Here's how the part is built. I have some questions about the finished solid (model axes, mm). Face numbers are marked on the shaded views. A direction names the side the tool comes from. Coordinates: 2 decimals unless noted, no trailing zeros. Order: outer loops, then holes, each group sorted by start corner. A loop starts at its lowest first (then second) coordinate and runs counter-clockwise, first axis right, second up. Notation, with made-up numbers: (77, 64.5) - (82, 64.5) arc R29 ccw to (82, 103.5) - close; hole circle Ø4 at (-9, -33). An arc over 180 degrees is marked (long way). Answer as CSV lines item,"result". Start each with the question number.
Q1. Suppose I cut it at D-D (y = -0.5). Please give me the cut outline in (x, z), then the cut area to 3 significant figures.
Q2. For the marked faces 1 and 2, which set-ups out of +Z, -Z, +X, -X, +Y, -Y let a thin tool reach every point of the face, with its end or its side?
Q3. For pin 1 Ø0.8 at (x, y) = (-17, 59.5) entering from +Z; pin 2 Ø4 at (x, z) = (33, 14) entering from +Y; pin 3 Ø2.5 at (y, z) = (60, -5) entering from +X, each with a flat end and sliding along its axis, tell me the tip position at first contact or that it passes through.
Q4. I need wall thicknesses on line 1 (X direction, y = 6, z = 3); line 2 (Z direction, x = -16, y = 4). Which ranges of each line are inside material? Lowest first, please.
Q5. Suppose I cut it at B-B (x = 18.3). Please give me the cut outline in (y, z), then the cut area to 3 significant figures.
Q6. Thinking about a two-plate mould opening in X: for the marked faces 3, 4 and 5, which applies, released by +X, released by -X, zero draft, split by the parting line, or undercut?
Q7. Suppose I cut it at A-A (z = 11.5). Please give me the cut outline in (x, y).
Q8. Suppose I cut it at C-C (z = -4). Please give me the cut outline in (x, y).
Autodesk Inventor part; units mm, degrees
ref_plane "YZ Plane" through (0, 0, 0) normal (1, 0, 0) x (0, 1, 0)
ref_plane "XZ Plane" through (0, 0, 0) normal (0, 1, 0) x (-1, 0, 0)
ref_plane "XY Plane" through (0, 0, 0) normal (0, 0, 1) x (1, 0, 0)
sketch "Sketch1" plane through (0, 0, 0) normal (0, 0, 1) x (1, 0, 0)
  line L0 (-42.25, 42.25) -> (42.25, 42.25)
  line L1 (42.25, 42.25) -> (42.25, -42.25)
  line L2 (42.25, -42.25) -> (-42.25, -42.25)
  line L3 (-42.25, -42.25) -> (-42.25, 42.25)
  line L4 (-42.25, 42.25) -> (42.25, -42.25) construction
  line L5 (42.25, 42.25) -> (-42.25, -42.25) construction
  line L6 (-45, 45) -> (45, 45)
  line L7 (45, 45) -> (45, -45)
  line L8 (45, -45) -> (-45, -45)
  line L9 (-45, -45) -> (-45, 45)
  line L10 (-45, 45) -> (45, -45) construction
  line L11 (45, 45) -> (-45, -45) construction
  point P0 (0, 0)
  dimension "d0" = 84.5
  dimension "d1" = 84.5
  dimension "d2" = 90
  dimension "d3" = 90
extrude "Extrusion1" add sketch "Sketch1" along normal blind 18
extrude "Extrusion2" add sketch "Sketch1" against normal blind 8 contours L0 L1 L2 L3 | L6 L7 L8 L9
sketch "Sketch2" plane through (0, 0, 18) normal (0, 0, 1) x (1, 0, 0)
  line L0 (42.25, -42.25) -> (42.25, 42.25)
  line L1 (42.25, 42.25) -> (-42.25, 42.25)
  line L2 (-42.25, 42.25) -> (-42.25, -42.25)
  line L3 (-42.25, -42.25) -> (42.25, -42.25)
  circle A0 centre (42.25, -42.25) radius 1.5
  line L4 (42.25, -42.25) -> (-42.25, -42.25)
  circle A1 centre (-42.25, -42.25) radius 1.5
  circle A2 centre (42.25, 42.25) radius 1.5
  line L5 (-42.25, 42.25) -> (42.25, 42.25)
  circle A3 centre (-42.25, 42.25) radius 1.5
  point P0 (0, 0)
  dimension "d8" = 3
  dimension "d9" = 3
  dimension "d10" = 3
  dimension "d11" = 3
extrude "Extrusion3" cut sketch "Sketch2" against normal up to surface (18 mm away) contours L3 A0 L0 | L0 A0 L3 | A2 L1 L0 | L0 L1 A2 | A1 L2 L3 | L3 L2 A1 | A3 L2 L1 | L1 L2 A3
sketch "Sketch3" plane through (42.25, -40.75, 0) normal (-1, 0, 0) x (0, 0, 1)
  line L0 (18, 81.5) -> (0, 81.5)
  line L1 (0, 0) -> (0, 81.5)
  line L2 (0, 0) -> (18, 0)
  line L3 (18, 81.5) -> (18, 0)
  line L4 (9.5, 56.5) -> (19.5, 56.5)
  line L5 (19.5, 56.5) -> (19.5, 45)
  line L6 (19.5, 45) -> (9.5, 45)
  line L7 (9.5, 45) -> (9.5, 56.5)
  point P0 (0, 40.75)
  dimension "d14" = 10
  dimension "d15" = 11.5
  dimension "d16" = 25
  dimension "d17" = 9.5
extrude "Extrusion4" cut sketch "Sketch3" against normal blind 10 contours L4 L5 L6 L3 | L3 L6 L7 L4
sketch "Sketch4" plane through (-40.75, 42.25, 0) normal (0, -1, 0) x (1, 0, 0)
  line L0 (0, 18) -> (0, 0)
  line L1 (81.5, 0) -> (0, 0)
  line L2 (81.5, 0) -> (81.5, 18)
  line L3 (0, 18) -> (81.5, 18)
  line L4 (0, 18) -> (81.5, 18)
  line L5 (81.5, 0) -> (0, 0)
  line L6 (45.75, 18) -> (35.75, 18)
  line L7 (35.75, 18) -> (35.75, 0)
  line L8 (35.75, 0) -> (45.75, 0)
  line L9 (45.75, 0) -> (45.75, 18)
  point P0 (40.75, 18)
  point P1 (40.75, 18)
  dimension "d22" = 10
extrude "Extrusion5" cut sketch "Sketch4" against normal up to surface (2.75 mm away) contours L3 L9 L1 L7
sketch "Sketch5" plane through (0, 0, -8) normal (0, 0, -1) x (-1, 0, 0)
  line L0 (45, 45) -> (-45, 45)
  line L1 (-45, 45) -> (-45, -45)
  line L2 (-45, -45) -> (45, -45)
  line L3 (45, -45) -> (45, 45)
  line L4 (-24, 45) -> (24, 45)
  line L5 (24, 45) -> (24, 75)
  line L6 (24, 75) -> (-24, 75)
  line L7 (-24, 75) -> (-24, 45)
  circle A0 centre (-15, 60) radius 1.3
  circle A1 centre (17, 60) radius 1.3
  point P0 (0, 0)
  point P1 (0, 45)
  point P2 (-24, 60)
  dimension "d25" = 48
  dimension "d26" = 30
  dimension "d27" = 2.6
  dimension "d28" = 2.6
  dimension "d29" = 32
extrude "Extrusion6" add sketch "Sketch5" against normal up to surface (8 mm away) contours L0 L7 L6 L5
extrude "Extrusion7" add sketch "Sketch5" against normal blind 13 contours A0 | A1
fillet "Fillet1" radius 10 4 edges at (24, 75, -4) (-24, 75, -4) (24, 45, -4) (-24, 45, -4)
fillet "Fillet2" radius 1.5 4 edges at (45, 45, 5) (-45, 45, 5) (45, -45, 5) (-45, -45, 5)
sketch "Sketch6" plane through (0, 0, -8) normal (0, 0, -1) x (-1, 0, 0)
  circle A0 centre (18.3, -5) radius 6.1
  circle A1 centre (6.1, -5) radius 6.1
  circle A2 centre (-6.1, -5) radius 6.1
  circle A3 centre (-18.3, -5) radius 6.1
  line L0 (-43.5, -45) -> (43.5, -45)
  point P0 (0, 0)
  point P1 (0, -5)
  point P2 (0, -45)
  dimension "d38" = 12.2
  dimension "d39" = 12.2
  dimension "d37" = 12.2
  dimension "d40" = 12.2
  dimension "d41" = 40
extrude "Extrusion8" cut sketch "Sketch6" against normal blind 1.6
properties part number "base"
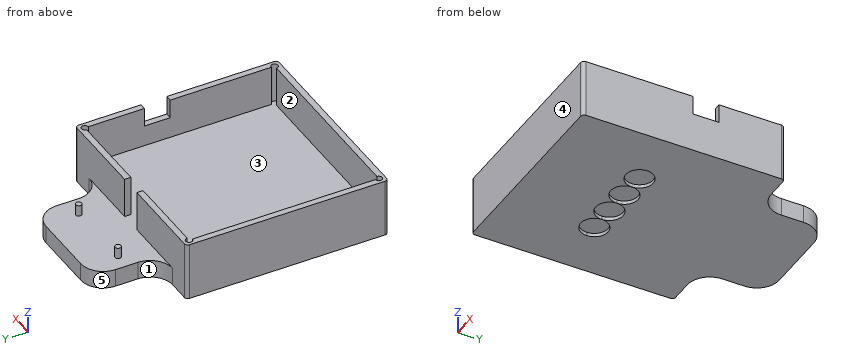
Here are the results:
1,outline,"(-45, -8) - (-22.42, -8) - (-22.42, -6.4) - (-14.18, -6.4) - (-14.18, -8) - (-10.22, -8) - (-10.22, -6.4) - (-1.98, -6.4) - (-1.98, -8) - (1.98, -8) - (1.98, -6.4) - (10.22, -6.4) - (10.22, -8) - (14.18, -8) - (14.18, -6.4) - (22.42, -6.4) - (22.42, -8) - (45, -8) - (45, 18) - (42.25, 18) - (42.25, 0) - (-42.25, 0) - (-42.25, 18) - (-45, 18) - close"
1,area,"766 mm²"
2,face 1,"+Z, -Z, -X, +Y"
2,face 2,"+Z"
3,pin 1,"stops at z = 5"
3,pin 2,"stops at y = 45"
3,pin 3,"stops at x = 24"
4,line 1,"x = -45 to -42.25, 42.25 to 45"
4,line 2,"z = -8 to 0"
5,outline,"(-45, -8) - (-11.1, -8) - (-11.1, -6.4) - (1.1, -6.4) - (1.1, -8) - (74.03, -8) - (74.03, 0) - (45, 0) - (45, 18) - (42.25, 18) - (42.25, 0) - (-42.25, 0) - (-42.25, 18) - (-45, 18) - close"
5,area,"1,030 mm²"
6,face 3,"undercut"
6,face 4,"zero draft"
6,face 5,"released by -X"
7,outline,"(-45, -43.5) arc R1.5 ccw to (-43.5, -45) - (43.5, -45) arc R1.5 ccw to (45, -43.5) - (45, 4.25) - (42.25, 4.25) - (42.25, -40.75) arc R1.5 cw (long way) to (40.75, -42.25) - (-40.75, -42.25) arc R1.5 cw (long way) to (-42.25, -40.75) - (-42.25, 40.75) arc R1.5 cw (long way) to (-40.75, 42.25) - (-5, 42.25) - (-5, 45) - (-43.5, 45) arc R1.5 ccw to (-45, 43.5) - close; (5, 42.25) - (40.75, 42.25) arc R1.5 cw (long way) to (42.25, 40.75) - (42.25, 15.75) - (45, 15.75) - (45, 43.5) arc R1.5 ccw to (43.5, 45) - (5, 45) - close"
8,outline,"(-45, -43.5) arc R1.5 ccw to (-43.5, -45) - (43.5, -45) arc R1.5 ccw to (45, -43.5) - (45, 43.5) arc R1.5 ccw to (43.5, 45) - (34, 45) arc R10 cw to (24, 55) - (24, 65) arc R10 ccw to (14, 75) - (-14, 75) arc R10 ccw to (-24, 65) - (-24, 55) arc R10 cw to (-34, 45) - (-43.5, 45) arc R1.5 ccw to (-45, 43.5) - close"
